from build123d import *

# Parameters (mm, degrees)
CYLINDER1994_R               = 1.5
CYLINDER1994_DEPTH           = 60
CYLINDER1991_R               = 1.5
CYLINDER1991_DEPTH           = 60
CYLINDER1992_R               = 1.5
CYLINDER1992_DEPTH           = 60
CYLINDER1993_R               = 1.5
CYLINDER1993_DEPTH           = 60
COMPOUND1074_PLACEMENT_ANGLE = 225
CYLINDER1990_R               = 3
CYLINDER1990_DEPTH           = 3
CYLINDER1987_R               = 3
CYLINDER1987_DEPTH           = 3
CYLINDER1988_R               = 3
CYLINDER1988_DEPTH           = 3
CYLINDER1989_R               = 3
CYLINDER1989_DEPTH           = 3
COMPOUND1075_PLACEMENT_ANGLE = 225
CYLINDER1986_R               = 74
CYLINDER1986_DEPTH           = 40
BOX985_W                     = 42
BOX985_H                     = 72
BOX985_DEPTH                 = 50
COMPOUND1072_PLACEMENT_ANGLE = 225
BOX986_W                     = 54
BOX986_H                     = 78
BOX986_DEPTH                 = 10
COMPOUND1073_PLACEMENT_ANGLE = 225
CHAMFER076_SIZE              = 3
CHAMFER077_SIZE              = 3


with BuildPart() as obj1:
    # Cylinder1994 → Cylinder1994 (new body)
    with BuildSketch(Plane(origin=(-24, 74, -80), x_dir=(1, 0, 0), z_dir=(0, 0, 1))):
        Circle(CYLINDER1994_R)
    extrude(amount=CYLINDER1994_DEPTH)


with BuildPart() as obj2:
    # Cylinder1991 → Cylinder1991 (new body)
    with BuildSketch(Plane(origin=(-15, 135, -80), x_dir=(1, 0, 0), z_dir=(0, 0, 1))):
        Circle(CYLINDER1991_R)
    extrude(amount=CYLINDER1991_DEPTH)


with BuildPart() as obj3:
    # Cylinder1992 → Cylinder1992 (new body)
    with BuildSketch(Plane(origin=(15, 135, -80), x_dir=(1, 0, 0), z_dir=(0, 0, 1))):
        Circle(CYLINDER1992_R)
    extrude(amount=CYLINDER1992_DEPTH)


with BuildPart() as compound1074:
    # Cylinder1993 → Cylinder1993 (new body)
    with BuildSketch(Plane(origin=(24, 74, -80), x_dir=(1, 0, 0), z_dir=(0, 0, 1))):
        Circle(CYLINDER1993_R)
    extrude(amount=CYLINDER1993_DEPTH)

    # Compound1074: union obj1, obj2, obj3
    add(obj1.part)
    add(obj2.part)
    add(obj3.part)


with BuildPart() as compound1074_1:
    # Compound1074 placement: moved
    add(compound1074.part.moved(Location((0, 0, 100))).rotate(Axis((0, 0, 100), (0, 0, 1)), COMPOUND1074_PLACEMENT_ANGLE))


with BuildPart() as obj4:
    # Cylinder1990 → Cylinder1990 (new body)
    with BuildSketch(Plane(origin=(-24, 74, -80), x_dir=(1, 0, 0), z_dir=(0, 0, 1))):
        Circle(CYLINDER1990_R)
    extrude(amount=CYLINDER1990_DEPTH)


with BuildPart() as obj5:
    # Cylinder1987 → Cylinder1987 (new body)
    with BuildSketch(Plane(origin=(-15, 135, -80), x_dir=(1, 0, 0), z_dir=(0, 0, 1))):
        Circle(CYLINDER1987_R)
    extrude(amount=CYLINDER1987_DEPTH)


with BuildPart() as obj6:
    # Cylinder1988 → Cylinder1988 (new body)
    with BuildSketch(Plane(origin=(15, 135, -80), x_dir=(1, 0, 0), z_dir=(0, 0, 1))):
        Circle(CYLINDER1988_R)
    extrude(amount=CYLINDER1988_DEPTH)


with BuildPart() as compound1075:
    # Cylinder1989 → Cylinder1989 (new body)
    with BuildSketch(Plane(origin=(24, 74, -80), x_dir=(1, 0, 0), z_dir=(0, 0, 1))):
        Circle(CYLINDER1989_R)
    extrude(amount=CYLINDER1989_DEPTH)

    # Compound1075: union obj4, obj5, obj6
    add(obj4.part)
    add(obj5.part)
    add(obj6.part)


with BuildPart() as compound1075_1:
    # Compound1075 placement: moved
    add(compound1075.part.moved(Location((0, 0, 135))).rotate(Axis((0, 0, 135), (0, 0, 1)), COMPOUND1075_PLACEMENT_ANGLE))


with BuildPart() as obj7:
    # Cylinder1986 → Cylinder1986 (new body)
    with BuildSketch(Plane.XY.offset(44)):
        Circle(CYLINDER1986_R)
    extrude(amount=CYLINDER1986_DEPTH)


with BuildPart() as compound1072:
    # Box985 → Box985 (new body)
    with BuildSketch(Plane(origin=(-21.001071, 60.005081, 31), x_dir=(1, 0, 0), z_dir=(0, 0, 1))):
        with Locations((21, 36)):
            Rectangle(BOX985_W, BOX985_H)
    extrude(amount=BOX985_DEPTH)


with BuildPart() as compound1072_1:
    # Compound1072 placement: moved
    add(compound1072.part.rotate(Axis((0, 0, 0), (0, 0, 1)), COMPOUND1072_PLACEMENT_ANGLE))


with BuildPart() as cut676:
    # Box986 → Box986 (new body)
    with BuildSketch(Plane(origin=(-27.004408, 59.99801, 75), x_dir=(1, 0, 0), z_dir=(0, 0, 1))):
        with Locations((27, 39)):
            Rectangle(BOX986_W, BOX986_H)
    extrude(amount=BOX986_DEPTH)


with BuildPart() as cut676_1:
    # Compound1073 placement: moved
    add(cut676.part.moved(Location((0, 0, -20))).rotate(Axis((0, 0, -20), (0, 0, 1)), COMPOUND1073_PLACEMENT_ANGLE))

    # Cut670: cut Compound1072
    add(compound1072_1.part, mode=Mode.SUBTRACT)

    # Cut671: cut obj7
    add(obj7.part, mode=Mode.SUBTRACT)

    # Chamfer076
    chamfer076_edges = [cut676_1.edges().sort_by_distance(p)[0] for p in [
        (116.674329, -78.484329, 60),
        (78.490563, -116.668095, 60),
    ]]
    chamfer(chamfer076_edges, length=CHAMFER076_SIZE)

    # Chamfer077
    chamfer077_edges = [cut676_1.edges().sort_by_distance(p)[0] for p in [
        (91.182683, -52.992683, 55),
        (114.553009, -78.484329, 55),
        (53.000139, -91.177671, 55),
        (78.490563, -114.546775, 55),
        (97.582446, -97.576212, 55),
    ]]
    chamfer(chamfer077_edges, length=CHAMFER077_SIZE)

    # Cut675: cut Compound1075
    add(compound1075_1.part, mode=Mode.SUBTRACT)

    # Cut676: cut Compound1074
    add(compound1074_1.part, mode=Mode.SUBTRACT)


solid = cut676_1.part
Could you check a few things on this model? Use its own coordinates, in mm. A direction names the side the tool comes from. Round coordinates to 2 decimals unless told otherwise and drop trailing zeros. Order: outer loops, then holes, each group sorted by start corner. A loop starts at its lowest first (then second) coordinate and runs counter-clockwise, first axis right, second up.
Q1. Imagine slicing it at B-B, the plane x = 75. List the corners of the cut face in (y, z) for me, then the cut area to 3 significant figures.
Geometry says:
outline: (-113.18, 58) - (-108.93, 55) - (-104.7, 55) - (-104.7, 65) - (-113.18, 65) - close; (-45.3, 55) - (-41.05, 55) - (-36.81, 58) - (-36.81, 65) - (-45.3, 65) - close
area: 157 mm2
Q2. I'm going to push flat-ended pins straight in: P1, Ø2.5, axis at x = 106.07, y = -84.85, coming from the +Z side; P2, Ø6, axis at x = 38.5, z = 56, coming from the +Y side; P3, Ø3, axis at x = 68.5, y = -35.5, coming from the -Z side; P4, Ø2, axis at x = 86.5, z = 59.5, coming from the +Y side. Where does each tip first touch, or does it pass through?
Geometry says:
P1: passes through
P2: stops at y = -65.2
P3: stops at z = 58
P4: stops at y = -47.31
Q3. Which directions (+Z, -Z, +X, -X, +Y, -Y) give clear straight access to the entire face, cutting with the end or side of a thin tool? Please do faces 1 (the face through (93.55, -93.133, 59.93)), 2 (the face through (70, -37, 58)), 3 (the face through (55.605, -91.691, 56.521)).
Geometry says:
face 1: +Z, -Z
face 2: -Z
face 3: -Z, -X, -Y
Q4. Imagine slicing it at A-A, the plane z = 56. List the corners of the cut face in (x, y) for me.
Geometry says:
outline: (31.58, -66.93) - (32.65, -68) arc R3 cw (long way) to (36.65, -72) - (77.2, -112.55) - (79.78, -112.55) - (83.56, -108.77) arc R3 cw to (82.61, -104.07) - (78.49, -108.19) - (35.33, -65.02) arc R74 cw to start; (65.02, -35.32) - (67.12, -37.42) arc R3 cw to (68.01, -32.65) - (66.93, -31.57) arc R74 cw to start; (67.23, -37.53) - (108.19, -78.49) - (104.07, -82.61) arc R3 cw to (108.77, -83.56) - (112.55, -79.78) - (112.55, -77.19) - (72.01, -36.64) arc R3 cw to start; (82.86, -103.82) arc R3 cw to (87.56, -104.77) - (104.77, -87.56) arc R3 cw to (103.82, -82.86) - close
Q5. Thinking about a two-plate mould opening in Y: for faces 4 (the face through (58, -90, 55)), 5 (the face through (96.681, -96.386, 56.521)), 6 (the face through (86.236, -103.404, 56.479)), which applies, released by +Y, released by -Y, zero draft, split by the parting line, or undercut?
Geometry says:
face 4: zero draft
face 5: released by -Y
face 6: undercut
Q6. Imagine slicing it at D-D, the plane x = 58. List the corners of the cut face in (y, z) for me.
Geometry says:
outline: (-96.18, 58) - (-91.93, 55) - (-87.7, 55) - (-87.7, 65) - (-96.18, 65) - close
Q7. Please list where these lines run through material, in increasing order: probe 1 along X at (y, z) = (-69, 59); probe 2 along Y at (x, z) = (69.5, 60.5); probe 3 along Y at (x, z) = (79, 60).
Geometry says:
probe 1: x = 30.82 to 33.88, 36.83 to 39.3, 98.7 to 107.19
probe 2: y = -107.68 to -99.2, -39.8 to -36.84, -33.87 to -31.31
probe 3: y = -114.55 to -107.68, -49.3 to -40.81
Q8. Imagine slicing it at C-C, the plane y = -98. List the corners of the cut face in (x, z) for me, then the cut area to 3 significant figures.
Geometry says:
outline: (59.82, 58) - (64.07, 55) - (68.3, 55) - (68.3, 65) - (59.82, 65) - close; (88.68, 55) - (92.92, 55) - (97.16, 58) - (97.16, 65) - (88.68, 65) - close
area: 157 mm2
